Design review of the part built by this model. Coordinates are the model's own, in mm. Face numbers are marked on the shaded views. Coordinates: 2 decimals unless noted, no trailing zeros. Write each loop counter-clockwise with the first axis right and the second up, starting at its lowest first coordinate (ties: lowest second). Pieces come first, ordered by that corner, then holes. Notation, with made-up numbers: (66, 63) - (119, 63) arc R27 ccw to (119, 81) - close; hole circle Ø6 at (20.5, 47.25). An arc over 180 degrees is marked (long way). One line per item, written item: value.
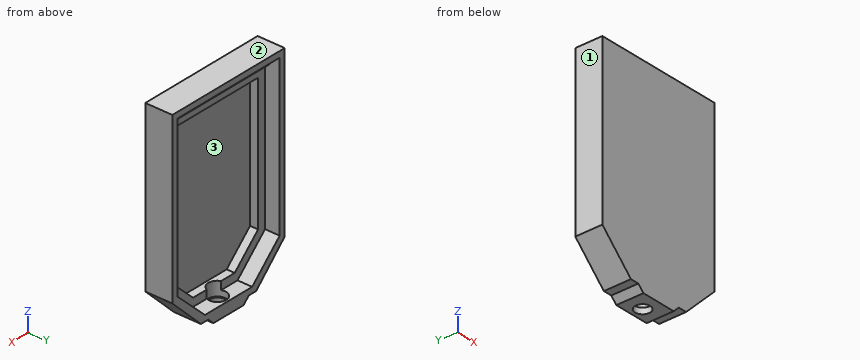
Autodesk Inventor part; units mm, degrees
ref_plane "YZ Plane" through (0, 0, 0) normal (1, 0, 0) x (0, 1, 0)
ref_plane "XZ Plane" through (0, 0, 0) normal (0, 1, 0) x (-1, 0, 0)
ref_plane "XY Plane" through (0, 0, 0) normal (0, 0, 1) x (1, 0, 0)
sketch "Náčrt1" plane through (0, 0, 0) normal (0, 1, 0) x (-1, 0, 0)
  line L0 (20, -19.5) -> (20, 29.85) construction
  line L1 (20, 29.85) -> (-20, 29.85) construction
  line L2 (-20, 29.85) -> (-20, -19.5) construction
  line L3 (-20, -19.5) -> (-9.25, -29.85) construction
  line L4 (-9.25, -29.85) -> (9.25, -29.85) construction
  line L5 (9.25, -29.85) -> (20, -19.5) construction
  line L6 (0, 0) -> (20, 29.85) construction
  line L7 (0, 0) -> (-20, 29.85) construction
  line L8 (0, 0) -> (-20, -29.85) construction
  line L9 (-20, -29.85) -> (-9.25, -29.85) construction
  line L10 (-20, -29.85) -> (-20, -19.5)
  line L11 (17.5, -18.4366) -> (17.5, 27.35)
  line L12 (17.5, 27.35) -> (-17.5, 27.35)
  line L13 (-17.5, 27.35) -> (-17.5, -18.4366)
  line L14 (-17.5, -18.4366) -> (-8.2421, -27.35)
  line L15 (-8.2421, -27.35) -> (8.2421, -27.35)
  line L16 (8.2421, -27.35) -> (17.5, -18.4366)
  line L17 (20.25, -19.6063) -> (20.25, 30.1)
  line L18 (20.25, 30.1) -> (-20.25, 30.1)
  line L19 (-20.25, 30.1) -> (-20.25, -19.6063)
  line L20 (-20.25, -19.6063) -> (-9.3508, -30.1)
  line L21 (-9.3508, -30.1) -> (9.3508, -30.1)
  line L22 (9.3508, -30.1) -> (20.25, -19.6063)
  line L23 (22.25, -20.7863) -> (22.25, 32.1)
  line L24 (22.25, 32.1) -> (-22.25, 32.1) construction
  line L25 (-22.25, 32.1) -> (-22.25, -20.7863)
  line L26 (-22.25, -20.7863) -> (-10.9363, -32.1)
  line L27 (-10.9363, -32.1) -> (10.9363, -32.1)
  line L28 (10.9363, -32.1) -> (22.25, -20.7863)
  line L29 (20.25, 30.1) -> (20.25, 34.1)
  line L30 (20.25, 34.1) -> (-20.25, 34.1)
  line L31 (-20.25, 34.1) -> (-20.25, 30.1)
  line L32 (22.25, 32.1) -> (22.25, 36.1)
  line L33 (22.25, 36.1) -> (-22.25, 36.1)
  line L34 (-22.25, 36.1) -> (-22.25, 32.1)
  line L35 (20.25, 30.7) -> (-20.25, 30.7)
  point P0 (0, -32.1)
  dimension "d0" = 40
  dimension "d1" = 59.7
  dimension "d2" = 18.5
  dimension "d4" = 49.35
  dimension "d6" = 2.5
  dimension "d9" = 4
  dimension "d10" = 2
  dimension "d19" = 0.25
  dimension "d20" = 2
  dimension "d21" = 135
  dimension "d22" = 2
  dimension "d24" = 16
  dimension "d45" = 0.6
extrude "Vysunutí1" add sketch "Náčrt1" along normal blind 1.5 contours L20 L19 L18 L17 L22 L21 | L26 L25 L34 L33 L32 L23 L28 L27 | L31 L35 L29 L18 | L31 L30 L29 L35 | L16 L15 L14 L13 L12 L11
extrude "Vysunutí2" add sketch "Náčrt1" along normal blind 4.25 contours L20 L19 L18 L17 L22 L21 | L31 L35 L29 L18
extrude "Vysunutí3" add sketch "Náčrt1" along normal blind 5.75 contours L31 L30 L29 L35
extrude "Vysunutí4" add sketch "Náčrt1" along normal blind 9.25 contours L26 L25 L34 L33 L32 L23 L28 L27
sketch "Náčrt2" plane through (0, 0, 0) normal (0, -1, 0) x (1, 0, 0)
  line L0 (10.9363, -32.1) -> (-10.9363, -32.1)
  line L1 (22.25, -20.7863) -> (10.9363, -32.1)
  line L2 (22.25, 36.1) -> (22.25, -20.7863)
  line L3 (-22.25, 36.1) -> (22.25, 36.1)
  line L4 (-22.25, -20.7863) -> (-22.25, 36.1)
  line L5 (-10.9363, -32.1) -> (-22.25, -20.7863)
  line L6 (8, -32.1) -> (6, -34.1)
  line L7 (6, -34.1) -> (-6, -34.1)
  line L8 (-6, -34.1) -> (-8, -32.1)
  line L9 (10.9363, -32.1) -> (-10.9363, -32.1)
  line L10 (10.9363, -32.1) -> (6, -34.1) construction
  line L11 (-6, -34.1) -> (-10.9363, -32.1) construction
  point P0 (0, 0)
  dimension "d25" = 45
  dimension "d26" = 2
  dimension "d27" = 12
extrude "Vysunutí5" add sketch "Náčrt2" against normal up to surface (9.25 mm away) contours L6 L7 L8 L0
sketch "Náčrt3" plane through (-9.3508, 4.25, -30.1) normal (0, 0, 1) x (1, 0, 0)
  line L0 (18.7016, 0) -> (0, 0)
  line L1 (18.7016, 0) -> (18.7016, 5)
  line L2 (0, 5) -> (18.7016, 5)
  line L3 (0, 0) -> (0, 5)
  line L4 (17.5929, -2.75) -> (1.1087, -2.75)
  line L5 (17.5929, -2.75) -> (17.5929, 0)
  line L6 (1.1087, 0) -> (17.5929, 0)
  line L7 (1.1087, -2.75) -> (1.1087, 0)
  circle A0 centre (9.3508, 1.175) radius 3.075
  line L8 (3.3508, 5) -> (15.3508, 5)
  line L9 (15.3508, -4.25) -> (15.3508, 5)
  line L10 (3.3508, -4.25) -> (15.3508, -4.25)
  line L11 (3.3508, -4.25) -> (3.3508, 5)
  line L12 (29.6008, 1.5) -> (-10.8992, 1.5)
  point P0 (9.3508, -4.25)
  point P1 (29.6008, 0.83)
  point P2 (-10.8992, 0.83)
  point P3 (9.3508, 5)
  point P4 (9.3508, 1.5)
  point P5 (9.3508, 5)
  point P6 (9.3508, 0)
  point P7 (9.3508, -2.75)
  point P8 (-10.8992, 1.5)
  dimension "d31" = 6.15
  dimension "d46" = 2.75
extrude "Vysunutí6" cut sketch "Náčrt3" along normal blind 7 and the other way blind 2 contours A0 L0 | L0 A0 L12 | L12 A0
sketch "Náčrt4" plane through (0, 5.425, -32.1) normal (0, 0, 1) x (1, 0, 0)
  circle A0 centre (0, 0) radius 3.075
  point P0 (0, -5.425)
  point P1 (-1.4433, 2.63)
  point P2 (1.4433, 2.63)
  point P3 (-1.199, 2.75)
  point P4 (1.199, 2.75)
hole "Díra1" at (0, 5.425, -32.1) direction (0, 0, -1) diameter 5.15 end through all
equation "\"d10\" = d8"
properties part number "rc5_box_2"
1. Consider section A-A, the plane x = 0. Write out the cut boundary in (y, z).
Answer block:
outline: (0, -34.1) - (2.85, -34.1) - (2.85, -32.1) - (2.35, -32.1) - (2.35, -27.35) - (1.5, -27.35) - (1.5, 27.35) - (4.25, 27.35) - (4.25, 30.7) - (5.75, 30.7) - (5.75, 34.1) - (9.25, 34.1) - (9.25, 36.1) - (0, 36.1) - close; (8, -34.1) - (9.25, -34.1) - (9.25, -30.1) - (8.5, -30.1) - (8.5, -32.1) - (8, -32.1) - close
2. Wall thickness on line 1 along X through (y, z) = (3.75, 0.5); line 2 along Z through (x, y) = (3.5, 3.5); line 3 along X through (y, z) = (5.75, -13.5): over which ranges is each line inside the solid? List them lowest first.
Answer block:
line 1: x = -22.25 to -17.5, 17.5 to 22.25
line 2: z = -34.1 to -27.35, 27.35 to 36.1
line 3: x = -22.25 to -20.25, 20.25 to 22.25
3. Mouldability with a two-part tool opening along Z and no side actions: class the marked faces 1, 2 and 3 as released by +Z, released by -Z, zero draft, split by the parting line, or undercut.
Answer block:
face 1: zero draft
face 2: released by +Z
face 3: undercut
4. Insertion check: pin 1 Ø10.5 at (x, z) = (-2.5, -10.5) entering from +Y; pin 2 Ø0.8 at (x, y) = (-8, 5) entering from -Z; pin 3 Ø2 at (x, y) = (-11.5, 5) entering from -Z. Each pin has a flat end and moves straight along its axis. Give the tip position at first contact, or say it passes through.
Answer block:
pin 1: stops at y = 1.5
pin 2: stops at z = -32.5
pin 3: stops at z = -32.1
5. Consider section B-B, the plane z = 5. Write out the cut boundary in (x, y).
Answer block:
outline: (-22.25, 0) - (22.25, 0) - (22.25, 9.25) - (20.25, 9.25) - (20.25, 4.25) - (17.5, 4.25) - (17.5, 1.5) - (-17.5, 1.5) - (-17.5, 4.25) - (-20.25, 4.25) - (-20.25, 9.25) - (-22.25, 9.25) - close
6. Consider section C-C, the plane y = 7. Write out the cut boundary in (x, z), then the cut area to 3 significant figures.
Answer block:
outline: (-22.25, -20.79) - (-10.94, -32.1) - (-8, -32.1) - (-6, -34.1) - (-2.04, -34.1) - (-2.04, -32.1) - (-2.64, -32.1) - (-2.64, -30.1) - (-9.35, -30.1) - (-20.25, -19.61) - (-20.25, 34.1) - (20.25, 34.1) - (20.25, -19.61) - (9.35, -30.1) - (2.64, -30.1) - (2.64, -32.1) - (2.04, -32.1) - (2.04, -34.1) - (6, -34.1) - (8, -32.1) - (10.94, -32.1) - (22.25, -20.79) - (22.25, 36.1) - (-22.25, 36.1) - close
area: 430 mm^2
